from build123d import *

# Parameters (mm, degrees)
SCHIZZO1_R                                           = 110
SCHIZZO1_R_2                                         = 55
ESTRUSIONE_ESTRUSIONE1_DEPTH                         = 20
SCHIZZO2_W                                           = 20
SCHIZZO2_H                                           = 11.25
RACCORDO1_R                                          = 2
SMUSSO1_SIZE                                         = 2
FORO_LAMATO_PER_VITE_M8_A_TESTA_CILINDRI_D           = 9
FORO_LAMATO_PER_VITE_M8_A_TESTA_CILINDRI_CBORE_D     = 15
FORO_LAMATO_PER_VITE_M8_A_TESTA_CILINDRI_CBORE_DEPTH = 8
RIPETIZIONECIRCOLARE1_COUNT                          = 4


with BuildPart() as part:
    # Schizzo1 → Estrusione-Estrusione1 (new body)
    with BuildSketch(Plane.XY):
        Circle(SCHIZZO1_R)
        Circle(SCHIZZO1_R_2, mode=Mode.SUBTRACT)
    extrude(amount=ESTRUSIONE_ESTRUSIONE1_DEPTH)

    # Schizzo2 → Rivoluzione1 (revolve)
    with BuildSketch(Plane(origin=(0, 0, 0), x_dir=(0, 0, -1), z_dir=(1, 0, 0)), mode=Mode.PRIVATE) as rivoluzione1_sk:
        with Locations((10, 73.125)):
            Rectangle(SCHIZZO2_W, SCHIZZO2_H)
    revolve(rivoluzione1_sk.sketch.rotate(Axis((0, 0, 0), (0, 0, -1)), 90), axis=Axis((0, 0, 0), (0, 0, -1)))

    # Raccordo1
    raccordo1_edges = [part.edges().sort_by_distance(p)[0] for p in [
        (-110, 0, 20),
    ]]
    fillet(raccordo1_edges, radius=RACCORDO1_R)

    # Smusso1
    smusso1_edges = [part.edges().sort_by_distance(p)[0] for p in [
        (-67.5, 0, -20),
    ]]
    chamfer(smusso1_edges, length=SMUSSO1_SIZE)

    # Foro lamato per Vite M8 a testa cilindrica piana-1 (through all)
    with Locations(Plane.XY.offset(20)):
        with Locations((-62.75572683, 62.75572683)):
            foro_lamato_per_vite_m8_a_testa_cilindri = CounterBoreHole(FORO_LAMATO_PER_VITE_M8_A_TESTA_CILINDRI_D / 2, FORO_LAMATO_PER_VITE_M8_A_TESTA_CILINDRI_CBORE_D / 2, FORO_LAMATO_PER_VITE_M8_A_TESTA_CILINDRI_CBORE_DEPTH)

    # RipetizioneCircolare1: Foro lamato per Vite M8 a testa cilindrica piana-1 ×4 about axis
    ripetizionecircolare1_axis = Axis((0, 0, 0), (0, 0, 1))
    for i in range(1, RIPETIZIONECIRCOLARE1_COUNT):
        add(foro_lamato_per_vite_m8_a_testa_cilindri.rotate(ripetizionecircolare1_axis, i * 360 / RIPETIZIONECIRCOLARE1_COUNT), mode=Mode.SUBTRACT)


solid = part.part
Can you work these out from the model? Positions are in its coordinate system, mm. A direction names the side the tool comes from. Give positions to 0.01 mm unless a question says otherwise; leave off trailing zeros. Loops run counter-clockwise (first coordinate to the right, second up) from the corner with the lowest first, then second, coordinate; pieces in that order, holes last. Notation, with made-up numbers: (40.25, -2.75) -> (99.25, -2.75) arc R13 ccw to (99.25, 13.25) -> close; hole circle Ø9 at (12.5, 9.25). An arc over 180 degrees is marked (long way). Write item = value, one per line.
1) Suppose I cut it at A-A on y = 0. Write out the boundary of the cut face in (x, z), then the cut area to 3 significant figures.
Check result:
outline = (-110, 0) -> (-78.75, 0) -> (-78.75, -20) -> (-69.5, -20) -> (-67.5, -18) -> (-67.5, 0) -> (-55, 0) -> (-55, 20) -> (-108, 20) arc R2 ccw to (-110, 18) -> close; (55, 0) -> (67.5, 0) -> (67.5, -18) -> (69.5, -20) -> (78.75, -20) -> (78.75, 0) -> (110, 0) -> (110, 18) arc R2 ccw to (108, 20) -> (55, 20) -> close
area = 2,640 mm2
2) For faces 1 (the cylindrical face through (56.1, 59.3, 16.1)), 2 (the flat face through (-55.3, 0.3, 0)), 3 (the cylindrical face through (-11.923, -53.692, 9.86)), which set-ups out of +Z, -Z, +X, -X, +Y, -Y let a thin tool reach every point of the face, with its end or its side?
Check result:
face_1 = +Z
face_2 = -Z
face_3 = +Z, -Z
3) Will these pins go through, and if not, where does the flat tip stop? pin 1 (19.5 mm diameter, centred on x = 62.76, y = 62.76, fed in from -Z); pin 2 (12 mm diameter, centred on x = 60, y = 62.5, fed in from +Z); pin 3 (14.5 mm diameter, centred on x = 62.76, y = -62.76, fed in from +Z); pin 4 (5 mm diameter, centred on x = -61.5, z = -5.5, fed in from +Y).
Check result:
pin_1 = 0
pin_2 = 20
pin_3 = 12
pin_4 = 52.16
4) Suppose I cut it at C-C on z = 4.5. Write out the boundary of the cut face in (x, y), then the cut area to 3 significant figures.
Check result:
outline = circle Ø220 at (0, 0); hole circle Ø9 at (-62.76, -62.76); hole circle Ø9 at (-62.76, 62.76); hole circle Ø110 at (0, 0); hole circle Ø9 at (62.76, -62.76); hole circle Ø9 at (62.76, 62.76)
area = 28,300 mm2
5) Thinking about a two-plate mould opening in X: for faces 4 (the cylindrical face through (66.55, 65.175, 5.916)), 5 (the cylindrical face through (-17.071, 76.877, -10.14)), 6 (the flat face through (-58, -63, 12)), which applies, released by +X, released by -X, zero draft, split by the parting line, or undercut?
Check result:
face_4 = undercut
face_5 = split by the parting line
face_6 = undercut
6) I need wall thicknesses on L1, parallel to Z at x = -39, y = -84.5; L2, parallel to Y at x = 0, z = -9; L3, parallel to X at y = 55, z = -2.5. Which ranges of each line are inside material? Lowest first, please. Write a range as from..to.
Check result:
L1 = 0..20
L2 = -78.75..-67.5, 67.5..78.75
L3 = -56.36..-39.13, 39.13..56.36
